Work out the finished part from the listing and answer in its coordinate system (mm). Face numbers are marked on the shaded views. A direction names the side the tool comes from. Round coordinates to 2 decimals unless told otherwise and drop trailing zeros. Loops run counter-clockwise (first coordinate to the right, second up) from the corner with the lowest first, then second, coordinate; pieces in that order, holes last. Notation, with made-up numbers: (-26, 5) -> (-7, 5) arc R18 ccw to (-7, 36) -> close; hole circle Ø3 at (43, -1). An arc over 180 degrees is marked (long way). Use one line per item in the form item = value.
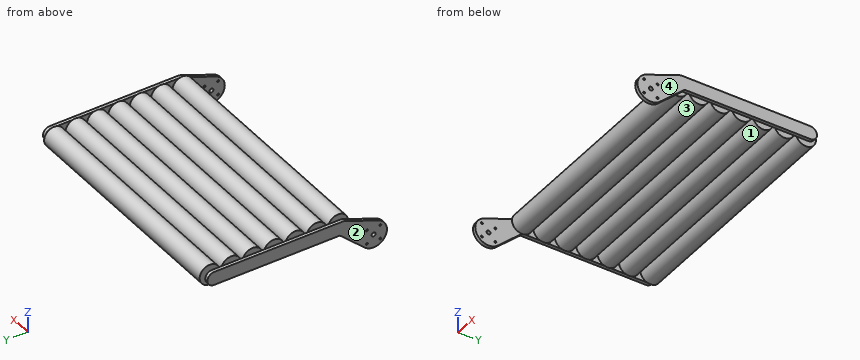
Autodesk Inventor part; units mm, degrees
ref_plane "Work Plane1" through (185, 0, 0) normal (1, 0, 0) x (0, 0, -1)
ref_plane "YZ Plane" through (0, 0, 0) normal (1, 0, 0) x (0, 1, 0)
ref_plane "XZ Plane" through (0, 0, 0) normal (0, 1, 0) x (-1, 0, 0)
sketch "Sketch1" plane through (0, 0, 0) normal (1, 0, 0) x (0, 1, 0)
  line L0 (-0.1455, -0.2526) -> (28.1388, 28.0317)
  line L1 (-0.1455, -0.2526) -> (39.8545, -0.2526) construction
  arc A0 (-7.3244, 18.4146) -> (13.2595, -15.0953) centre (-0.1455, -0.2526) ccw
  line L2 (26.5, 28.4) -> (87.1548, 28.4)
  line L3 (26.5, 28.4) -> (46.5, 28.4) construction
  circle A1 centre (46.5, 28.4) radius 15 construction
  circle A2 centre (78.5, 28.4) radius 15 construction
  circle A3 centre (110.5, 28.4) radius 15 construction
  circle A4 centre (142.5, 28.4) radius 15 construction
  circle A5 centre (174.5, 28.4) radius 15 construction
  line L4 (174.5, 28.4) -> (46.5, 28.4) construction
  line L5 (174.5, 38.4) -> (46.5, 38.4)
  line L6 (50.3473, 18.4) -> (174.5, 18.4)
  arc A6 (46.5, 38.4) -> (46.5, 18.4) centre (46.5, 28.4) ccw construction
  line L7 (13.2595, -15.0953) -> (50.3473, 18.4)
  line L8 (-7.3244, 18.4146) -> (42.9106, 37.7336)
  arc A7 (46.5, 18.4) -> (53.2025, 20.9786) centre (46.5, 28.4) ccw construction
  arc A8 (46.5, 38.4) -> (42.9106, 37.7336) centre (46.5, 28.4) ccw
  circle A9 centre (46.5, 28.4) radius 2.5
  circle A10 centre (78.5, 28.4) radius 2.5
  circle A11 centre (110.5, 28.4) radius 2.5
  circle A12 centre (142.5, 28.4) radius 2.5
  circle A13 centre (174.5, 28.4) radius 2.5
  circle A14 centre (206.5, 28.4) radius 2.5
  circle A15 centre (238.5, 28.4) radius 2.5
  circle A16 centre (206.5, 28.4) radius 15 construction
  circle A17 centre (238.5, 28.4) radius 15 construction
  line L9 (174.5, 28.4) -> (238.5, 28.4) construction
  line L10 (174.5, 38.4) -> (238.5, 38.4)
  line L11 (238.5, 18.4) -> (174.5, 18.4)
  arc A18 (238.5, 18.4) -> (238.5, 38.4) centre (238.5, 28.4) ccw
  line L12 (-0.1455, -0.2526) -> (-10.1789, -10.7207) construction
  line L13 (-0.1455, -0.2526) -> (9.8879, -10.7207) construction
  line L14 (-0.1455, -0.2526) -> (-10.1789, 10.2155) construction
  line L15 (-0.1455, -0.2526) -> (9.8879, 10.2155) construction
  circle A19 centre (-10.1789, -10.7207) radius 1.5
  circle A20 centre (9.8879, -10.7207) radius 1.5
  circle A21 centre (-10.1789, 10.2155) radius 1.5
  circle A22 centre (9.8879, 10.2155) radius 1.5
  circle A23 centre (-0.1455, -0.2526) radius 3
  point P0 (0, 0)
  point P1 (110.5, 28.4)
  dimension "d4" = 40
  dimension "d5" = 45
  dimension "d9" = 20
  dimension "d10" = 32
  dimension "d11" = 20
  dimension "d13" = 5
  dimension "d16" = 32
  dimension "d38" = 20
  dimension "d39" = 14.5
  dimension "d40" = 14.5
  dimension "d41" = 3
  dimension "d42" = 6
extrude "Extrusion1" add sketch "Sketch1" along normal blind 5 contours L8 A8 L5 L10 A18 L11 L6 L7 A0 | A9 L2 | A10 L2 | L2 A10 | L2 A9 | A11 | A12 | A13 | A14 | A15
sketch "Sketch2" plane through (5, 0, 0) normal (1, 0, 0) x (0, 0, -1)
  circle A0 centre (-28.4, 46.5) radius 2.5
  circle A1 centre (-28.4, 238.5) radius 2.5
  circle A2 centre (-28.4, 46.5) radius 2.5
  circle A3 centre (-28.4, 238.5) radius 2.5
  line L0 (-28.4, 46.5) -> (-28.4, 238.5) construction
  line L1 (-13.4, 46.5) -> (-13.4, 238.5)
  line L2 (-43.4, 238.5) -> (-43.4, 46.5)
  arc A4 (-43.4, 46.5) -> (-13.4, 46.5) centre (-28.4, 46.5) ccw
  arc A5 (-13.4, 238.5) -> (-43.4, 238.5) centre (-28.4, 238.5) ccw
  circle A6 centre (-28.4, 206.5) radius 2.5
  circle A7 centre (-28.4, 174.5) radius 2.5
  circle A8 centre (-28.4, 142.5) radius 2.5
  circle A9 centre (-28.4, 110.5) radius 2.5
  circle A10 centre (-28.4, 78.5) radius 2.5
  point P0 (0, 0)
  dimension "d27" = 30
extrude "Extrusion2" add sketch "Sketch2" along normal blind 5 contours A0 | A1 | A6 | A7 | A8 | A9 | A10
sketch "Sketch3" plane through (10, 238.5, 28.4) normal (1, 0, 0) x (0, 0, -1)
  circle A0 centre (0, 0) radius 2.5
  circle A1 centre (0, 0) radius 15
  line L0 (0, 0) -> (0, -15) construction
  circle A2 centre (0, -32) radius 15
  circle A3 centre (0, -64) radius 15
  circle A4 centre (0, -96) radius 15
  circle A5 centre (0, -128) radius 15
  circle A6 centre (0, -160) radius 15
  circle A7 centre (0, -192) radius 15
  point P0 (28.4, -238.5)
  point P1 (0, -47)
  point P2 (0, -79)
  point P3 (0, -111)
  point P4 (0, -143)
  point P5 (0, -175)
  point P6 (0, -207)
  dimension "d28" = 30
  dimension "d31" = 32
extrude "Extrusion3" add sketch "Sketch3" along normal blind 175 contours A0 | A1 | A2 | A3 | A4 | A5 | A6 | A7
ref_plane "Work Plane1" through (185, 0, 0) normal (1, 0, 0) x (0, 0, -1)
mirror "Mirror2" about plane through (185, 0, 0) normal (1, 0, 0) of "Extrusion1", "Extrusion2", "Extrusion3"
properties part number "Orienter"
(1) Consider L1, parallel to X at y = 155, z = 32; L2, parallel to X at y = 96, z = 20; L3, parallel to X at y = 178.5, z = 15. Determine where each line is inside the solid, lowest interval first.
Completed:
L1 = 0 to 5, 10 to 360, 365 to 370
L2 = 0 to 5, 365 to 370
L3 = 10 to 360
(2) Find section B-B, the plane y = 132.5. Write down the section's boundary in (x, z), then the cut area to 3 significant figures.
Completed:
outline = (0, 18.4) -> (5, 18.4) -> (5, 38.4) -> (0, 38.4) -> close; (10, 17.22) -> (360, 17.22) -> (360, 39.58) -> (10, 39.58) -> close; (365, 18.4) -> (370, 18.4) -> (370, 38.4) -> (365, 38.4) -> close
area = 8,030 mm2
(3) Find section A-A, the plane x = 253. Write down the section's boundary in (y, z).
Completed:
outline = circle Ø30 at (46.5, 28.4); circle Ø30 at (78.5, 28.4); circle Ø30 at (110.5, 28.4); circle Ø30 at (142.5, 28.4); circle Ø30 at (174.5, 28.4); circle Ø30 at (206.5, 28.4); circle Ø30 at (238.5, 28.4)
(4) For the marked faces 1 and 2, determine the directions among +Z, -Z, +X, -X, +Y, -Y from which every point of the face is accessible in a straight line to the end or side of a thin tool.
Completed:
face_1 = none
face_2 = +Z, -Z, -X, +Y, -Y
(5) Given P1, Ø1, axis at x = 109.5, y = 49.5, coming from the +Z side; P2, Ø6, axis at x = 132, z = 20, coming from the +Y side; P3, Ø5.5, axis at x = 366.5, y = 133, coming from the +Z side; P4, Ø1.8, axis at y = 9.89, z = -10.72, coming from the +X side, each flat-ended and moving along its own axis, determine where each tip first touches the part or whether it passes through.
Completed:
P1 = 43.19
P2 = 252.49
P3 = 38.4
P4 = through
(6) For a pull along Y with two mould halves and no side action, classify the marked faces 3 and 4 as +Y half, -Y half, draft (parallel to the pull), parting line (faces both ways), or undercut.
Completed:
face_3 = undercut
face_4 = draft
